Autodesk Inventor part; units mm, degrees
ref_plane "YZ Plane" through (0, 0, 0) normal (1, 0, 0) x (0, 1, 0)
ref_plane "XZ Plane" through (0, 0, 0) normal (0, 1, 0) x (-1, 0, 0)
ref_plane "XY Plane" through (0, 0, 0) normal (0, 0, 1) x (1, 0, 0)
sketch "Skizze1" plane through (0, 0, 0) normal (0, 0, 1) x (1, 0, 0)
  line L0 (-25, 25) -> (25, 25)
  line L1 (25, 25) -> (25, -25)
  line L2 (25, -25) -> (-25, -25)
  line L3 (-25, -25) -> (-25, 25)
  point P0 (0, 0)
  point P1 (25, 0)
  point P2 (0, 25)
  dimension "d0" = 50
  dimension "d1" = 50
extrude "Extrusion1" add sketch "Skizze1" along normal blind 15
ref_plane "Arbeitsebene1" through (0, 0, 13) normal (0, 0, 1) x (1, 0, 0)
sketch "Skizze4" plane through (0, 0, 13) normal (0, 0, 1) x (1, 0, 0)
  circle A0 centre (-12.5, -12.5) radius 7.5
  line L0 (-25, 25) -> (-25, -25)
  circle A1 centre (12.5, -12.5) radius 7.5
  line L1 (25, -25) -> (25, 25)
  line L2 (-25, -25) -> (25, -25)
  circle A2 centre (-12.5, 12.5) radius 7.5
  line L3 (25, 25) -> (-25, 25)
  circle A3 centre (12.5, 12.5) radius 7.5
  point P0 (0, 0)
  dimension "d6" = 15
  dimension "d7" = 12.5
  dimension "d8" = 15
  dimension "d9" = 12.5
  dimension "d10" = 12.5
  dimension "d11" = 12.5
  dimension "d12" = 15
  dimension "d13" = 12.5
  dimension "d14" = 12.5
  dimension "d15" = 15
extrude "Extrusion2" cut sketch "Skizze4" against normal blind 8 contours A0 | A1 | A2 | A3
sketch "Skizze6" plane through (0, 0, 15) normal (0, 0, 1) x (1, 0, 0)
  circle A0 centre (-12.5, 0) radius 2.5
  circle A1 centre (0, 12.5) radius 2.5
  circle A2 centre (12.5, 0) radius 2.5
  circle A3 centre (0, -12.5) radius 2.5
  line L0 (25, 25) -> (-25, 25)
  line L1 (-25, 25) -> (-25, -25)
  line L2 (25, -25) -> (25, 25)
  point P0 (0, 0)
  dimension "d18" = 5
  dimension "d19" = 12.5
  dimension "d20" = 25
  dimension "d21" = 5
  dimension "d22" = 12.5
  dimension "d23" = 25
  dimension "d24" = 5
  dimension "d25" = 12.5
  dimension "d26" = 25
  dimension "d27" = 5
  dimension "d28" = 12.5
  dimension "d29" = 25
extrude "Extrusion3" cut sketch "Skizze6" against normal blind 10
sketch "Skizze7" plane through (0, 0, 0) normal (0, 0, -1) x (-1, 0, 0)
  circle A0 centre (0, 12.5) radius 2.5
  circle A1 centre (0, 12.5) radius 1
  circle A2 centre (0, -12.5) radius 2.5
  circle A3 centre (0, -12.5) radius 1
  circle A4 centre (-12.5, 0) radius 2.5
  circle A5 centre (-12.5, 0) radius 1
  circle A6 centre (12.5, 0) radius 2.5
  circle A7 centre (12.5, 0) radius 1
  point P0 (0, 0)
  dimension "d32" = 2
  dimension "d33" = 2
  dimension "d34" = 2
  dimension "d35" = 2
extrude "Extrusion4" cut sketch "Skizze7" against normal blind 10 contours A1 | A3 | A5 | A7
properties part number "TestBauteil"
Could you check a few things on this model? Use its own coordinates, in mm. A direction names the side the tool comes from. Round coordinates to 2 decimals unless told otherwise and drop trailing zeros. Write each loop counter-clockwise with the first axis right and the second up, starting at its lowest first coordinate (ties: lowest second). Pieces come first, ordered by that corner, then holes. Notation, with made-up numbers: M 5,2.5 L 9,2.5 A32 cw 9,35.5 Z; hole C 83.25,1.25 d9. An arc over 180 degrees is marked long. Write each question's results on one line, items separated by ' | '. Start each with the question number.
1. On a 3-axis mill with a long thin cutter (end or side, diameter ignored), from which of +Z, -Z, +X, -X, +Y, -Y can I reach the whole of each face in a straight line? I mean faces 5 (the face through (-13, 13, 13)), 6 (the face through (10, 0, 10)), 7 (the face through (25, 0, 7)). Say none if no direction works.
2. Thinking about a two-plate mould opening in Z: for faces 1 (the face through (0, -25, 7)), 2 (the face through (12, -12, 5)), 3 (the face through (-13, -12, 13)), 4 (the face through (0, 11, 5)), which applies, +Z half, -Z half, draft (parallel to the pull), parting line (faces both ways), or undercut?
3. Imagine slicing it at D-D on y = -18.5. List the corners of the cut face in (x, z) for me, and give its area (3 significant figures).
4. I need wall thicknesses on L1, parallel to Y at x = -12.5, z = 10; L2, parallel to Z at x = -16, y = 7; L3, parallel to Y at x = 8, z = 6.25. Which ranges of each line are inside material? Lowest first, please. Write a range as from..to.
5. I'm going to push a flat-ended pin straight in: pin 1 Ø1.2 at (x, y) = (0, 12.5) entering from -Z. Where does the tip first touch, or does it pass through?
6. Imagine slicing it at A-A on y = -12.5. List the corners of the cut face in (x, z) for me, and give its area (3 significant figures).
7. Imagine slicing it at C-C on y = 0. List the corners of the cut face in (x, z) for me, and give its area (3 significant figures).
Result sheet:
1) face 5: none | face 6: +Z | face 7: +Z, -Z, +X, +Y, -Y
2) face 1: draft | face 2: undercut | face 3: undercut | face 4: +Z half
3) outline: M -25,0 L 25,0 L 25,15 L -25,15 Z; hole M -17,5 L -8,5 L -8,13 L -17,13 Z; hole M 8,5 L 17,5 L 17,13 L 8,13 Z | area: 606 mm^2
4) L1: y = -25..-20, -5..-2.5, 2.5..5, 20..25 | L2: z = 0..5, 13..15 | L3: y = -25..-18.5, -6.5..6.5, 18.5..25
5) pin 1: passes through
6) outline: M -25,0 L -1,0 L -1,5 L -2.5,5 L -2.5,15 L -25,15 Z; M 1,0 L 25,0 L 25,15 L 2.5,15 L 2.5,5 L 1,5 Z; hole M -20,5 L -5,5 L -5,13 L -20,13 Z; hole M 5,5 L 20,5 L 20,13 L 5,13 Z | area: 450 mm^2
7) outline: M -25,0 L -13.5,0 L -13.5,5 L -15,5 L -15,15 L -25,15 Z; M -11.5,0 L 11.5,0 L 11.5,5 L 10,5 L 10,15 L -10,15 L -10,5 L -11.5,5 Z; M 13.5,0 L 25,0 L 25,15 L 15,15 L 15,5 L 13.5,5 Z | area: 630 mm^2
